Design review of the part built by this model. Coordinates are the model's own, in mm. A direction names the side the tool comes from. Round coordinates to 2 decimals unless told otherwise and drop trailing zeros. Loops run counter-clockwise (first coordinate to the right, second up) from the corner with the lowest first, then second, coordinate; pieces in that order, holes last. Notation, with made-up numbers: (-21, -6) -> (7, -6) arc R8 ccw to (7, -1) -> close; hole circle Ø10 at (-39, -13.5). An arc over 180 degrees is marked (long way). Answer as CSV lines item,"result". Start each with the question number.
(1) To check wall thickness, follow line 1 (Y direction, x = -19.5, z = 1.5); line 2 (X direction, y = -46, z = 4.75); line 3 (Y direction, x = -1.5, z = 4.25). State the ranges of each line that lie inside material, in increasing order. Write a range as from..to.
(2) Draft analysis for pull direction X (two halves, no side actions). For faces 1 (the face through (-50.8, 1, 3)), 2 (the face through (18.28, -6.34, 3.13)), 3 (the face through (-1, -50.8, 3)), state which applies: +X half, -X half, draft (parallel to the pull), parting line (faces both ways), or undercut.
(3) Take a section at B-B, the plane y = -2.87. Write out the cut boundary in (x, z), and give its area (3 significant figures).
(4) Take a section at A-A, the plane x = 19.05. Write out the cut boundary in (y, z).
(5) Machinability: for faces 4 (the face through (49.351, 49.272, 3.131)), 5 (the face through (-11.35, -30, 3)), which of the approach directions +Z, -Z, +X, -X, +Y, -Y give a long, thin tool a straight path to every point of the face, cutting with its end or side? Answer none if there is none.
(6) Take a section at D-D, the plane y = -24. Write out the cut boundary in (x, z).
(7) For P1, Ø3, axis at x = 3, y = 8.5, coming from the -Z side; P2, Ø1.5, axis at x = -7.5, y = -33, coming from the -Z side, all flat-tipped, find the tip position at first contact; note any pin that passes through.
(8) Take a section at C-C, the plane x = -34. Write out the cut boundary in (y, z).
from build123d import *

# Parameters (mm, degrees)
F0_R     = 2.2225
F0_R_2   = 3.556
F0_R_3   = 1.3
F0_W     = 72
F0_H     = 27
F1_DEPTH = 6.35


with BuildPart() as f1:
    # F0 (on Top) → F1 (new body)
    with BuildSketch(Plane.XY):
        with BuildLine():
            Line((45.72, 50.8), (-45.72, 50.8))
            ThreePointArc((-45.72, 50.8), (-49.312102, 49.312102), (-50.8, 45.72))
            Line((-50.8, 45.72), (-50.8, -45.72))
            ThreePointArc((-50.8, -45.72), (-49.312102, -49.312102), (-45.72, -50.8))
            Line((-45.72, -50.8), (45.72, -50.8))
            ThreePointArc((45.72, -50.8), (49.312102, -49.312102), (50.8, -45.72))
            Line((50.8, -45.72), (50.8, 45.72))
            ThreePointArc((50.8, 45.72), (49.312102, 49.312102), (45.72, 50.8))
        make_face()
        with Locations((-46.0375, -46.0375)):
            Circle(F0_R, mode=Mode.SUBTRACT)
        with BuildLine():
            ThreePointArc((-2, -40.022667), (-7.209059, -37.044447), (-9.68775, -31.58))
            Line((-9.68775, -31.58), (-11.35, -31.58))
            Line((-11.35, -31.58), (-11.35, -30.48))
            Line((-11.35, -30.48), (-11.35, -29.38))
            Line((-11.35, -29.38), (-9.68775, -29.38))
            ThreePointArc((-9.68775, -29.38), (-7.209059, -23.915553), (-2, -20.937333))
            Line((-2, -20.937333), (-2, -19.73))
            Line((-2, -19.73), (2, -19.73))
            Line((2, -19.73), (2, -20.937333))
            ThreePointArc((2, -20.937333), (9.75, -30.48), (2, -40.022667))
            Line((2, -40.022667), (2, -41.23))
            Line((2, -41.23), (-2, -41.23))
            Line((-2, -41.23), (-2, -40.022667))
        make_face(mode=Mode.SUBTRACT)
        with Locations((-19.05, -2.87)):
            Circle(F0_R_2, mode=Mode.SUBTRACT)
        with Locations((46.0375, -46.0375)):
            Circle(F0_R, mode=Mode.SUBTRACT)
        with Locations((19.05, -2.87)):
            Circle(F0_R_2, mode=Mode.SUBTRACT)
        with Locations((-37.5, 6.86)):
            Circle(F0_R_3, mode=Mode.SUBTRACT)
        with Locations((0, 22.06)):
            Rectangle(F0_W, F0_H, mode=Mode.SUBTRACT)
        with Locations((-37.5, 37.86)):
            Circle(F0_R_3, mode=Mode.SUBTRACT)
        with Locations((-46.0375, 46.0375)):
            Circle(F0_R, mode=Mode.SUBTRACT)
        with Locations((37.5, 6.86)):
            Circle(F0_R_3, mode=Mode.SUBTRACT)
        with Locations((37.5, 37.86)):
            Circle(F0_R_3, mode=Mode.SUBTRACT)
        with Locations((46.0375, 46.0375)):
            Circle(F0_R, mode=Mode.SUBTRACT)
    extrude(amount=F1_DEPTH)


solid = f1.part
The answers:
1,line 1,"-50.8..-6.4, 0.66..8.56, 35.56..50.8"
1,line 2,"-50.79..-48.26, -43.82..43.82, 48.26..50.79"
1,line 3,"-50.8..-41.23, -19.73..8.56, 35.56..50.8"
2,face 1,"-X half"
2,face 2,"undercut"
2,face 3,"draft"
3,outline,"(-50.8, 0) -> (-22.61, 0) -> (-22.61, 6.35) -> (-50.8, 6.35) -> close; (-15.49, 0) -> (15.49, 0) -> (15.49, 6.35) -> (-15.49, 6.35) -> close; (22.61, 0) -> (50.8, 0) -> (50.8, 6.35) -> (22.61, 6.35) -> close"
3,area,"555 mm²"
4,outline,"(-50.8, 0) -> (-6.43, 0) -> (-6.43, 6.35) -> (-50.8, 6.35) -> close; (0.69, 0) -> (8.56, 0) -> (8.56, 6.35) -> (0.69, 6.35) -> close; (35.56, 0) -> (50.8, 0) -> (50.8, 6.35) -> (35.56, 6.35) -> close"
5,face 4,"+Z, -Z, +X, +Y"
5,face 5,"+Z, -Z"
6,outline,"(-50.8, 0) -> (-7.29, 0) -> (-7.29, 6.35) -> (-50.8, 6.35) -> close; (7.29, 0) -> (50.8, 0) -> (50.8, 6.35) -> (7.29, 6.35) -> close"
7,P1,"z = 0"
7,P2,"through"
8,outline,"(-50.8, 0) -> (8.56, 0) -> (8.56, 6.35) -> (-50.8, 6.35) -> close; (35.56, 0) -> (50.8, 0) -> (50.8, 6.35) -> (35.56, 6.35) -> close"
